Part model, mm, in its own coordinate system. A direction names the side the tool comes from. Give positions to 0.01 mm unless a question says otherwise; leave off trailing zeros. Write each loop counter-clockwise with the first axis right and the second up, starting at its lowest first coordinate (ties: lowest second). Pieces come first, ordered by that corner, then holes. Notation, with made-up numbers: (20.25, 0) - (26.25, 0) arc R23 ccw to (26.25, 37) - close; hole circle Ø9 at (14, 65). An arc over 180 degrees is marked (long way). Answer as a JSON object with one key per item and string values. Group by question number.
```python
from build123d import *

# Parameters (mm, degrees)
CHANFREIN1_SIZE = 0.5


with BuildPart() as part:
    # Esquisse1 → Révolution1 (revolve)
    with BuildSketch(Plane(origin=(0, 0, 0), x_dir=(0, 0, -1), z_dir=(1, 0, 0))):
        Polygon((15.742003569, 4.5), (3.980428295, 2), (-1.019571705, 2), (-15.742003569, 10.5), (-15.742003569, 12), (-3.757996431, 12), (-3.757996431, 10), (-2.257996431, 10), (-2.257996431, 7), (15.742003569, 7), align=None)
    revolve(axis=Axis((0, 0, 15.742003569), (0, 0, -1)))

    # Chanfrein1
    chanfrein1_edges = [part.edges().sort_by_distance(p)[0] for p in [
        (0, -12, 15.742003569),
    ]]
    chamfer(chanfrein1_edges, length=CHANFREIN1_SIZE)


solid = part.part
```
1) Mould opens along X. For faces 1 (the flat face through (-3.4, -10.2, 15.742)), 2 (the cylindrical face through (-9.76, -2.17, 3)), 3 (the conical face through (-4.3, -1, 5.2)) say: pulls with the +X half, pulls with the -X half, needs draft (parallel to the pull), parting line crosses it, or undercut.
2) Drop flat-ended pins along their axis: P1, Ø12, axis at x = 9, z = 2, coming from the +Y side; P2, Ø4, axis at y = 3, z = -6.5, coming from the -X side; P3, Ø5, axis at x = -7.5, z = 11.5, coming from the -Y side. Give the stop position or say it passes through.
3) Band-saw the part on A-A (y = 0). List the corners of the cut face in (x, z), plus the area to 3 significant figures.
4) Which spindle directions (+Z, -Z, +X, -X, +Y, -Y) get a long thin tool onto all of the face, cutting with end or side? Do faces 4 (the flat face through (-5, 0, -15.742)), 5 (the cylindrical face through (-2.681, 6.466, -6.868)). Say none if no direction does.
5) Probe line 1 (X direction, y = 0, z = -1.8); line 2 (Y direction, x = 1, z = 12); line 3 (Y direction, x = -2, z = 10). List the from-to ranges inside material, lowest first.
6) Band-saw the part on D-D (z = 10). List the corners of the cut face in (x, y), plus the area to 3 significant figures.
7) Band-saw the part on C-C (z = -8). List the corners of the cut face in (x, y), plus the area to 3 significant figures.
Verdict:
{
 "1": {"face 1": "needs draft", "face 2": "parting line crosses it", "face 3": "undercut"},
 "2": {"P1": "y = 11.55", "P2": "x = -6.93", "P3": "y = -10.91"},
 "3": {"outline": "(-12, 3.76) - (-10, 3.76) - (-10, 2.26) - (-7, 2.26) - (-7, -15.74) - (-4.5, -15.74) - (-2, -3.98) - (-2, 1.02) - (-10.5, 15.74) - (-11.5, 15.74) - (-12, 15.24) - close; (2, -3.98) - (4.5, -15.74) - (7, -15.74) - (7, 2.26) - (10, 2.26) - (10, 3.76) - (12, 3.76) - (12, 15.24) - (11.5, 15.74) - (10.5, 15.74) - (2, 1.02) - close", "area": "289 mm2"},
 "4": {"face 4": "-Z, +X, -X, +Y, -Y", "face 5": "-Z"},
 "5": {"line 1": "-7 to -2, 2 to 7", "line 2": "-11.96 to -8.28, 8.28 to 11.96", "line 3": "-11.83 to -6.9, 6.9 to 11.83"},
 "6": {"outline": "circle Ø24 at (0, 0); hole circle Ø14.37 at (0, 0)", "area": "290 mm2"},
 "7": {"outline": "circle Ø14 at (0, 0); hole circle Ø5.71 at (0, 0)", "area": "128 mm2"}
}
